Part model, mm, in its own coordinate system. Coordinates: 2 decimals unless noted, no trailing zeros. Write each loop counter-clockwise with the first axis right and the second up, starting at its lowest first coordinate (ties: lowest second). Pieces come first, ordered by that corner, then holes. Notation, with made-up numbers: (65, -23) -> (71, -23) arc R27 cw to (71, 0) -> close; hole circle Ø2 at (75.5, 1.25). An arc over 180 degrees is marked (long way). One line per question, with ' | ' between items. Start each with the question number.
Item 1: Two-plate mould, pull along X, no slides. Class faces 1 (the flat face through (-1, 6, 5)), 2 (the flat face through (-29.739, -1, 2)), 3 (the cylindrical face through (5.31, -0.76, 2.46)): pulls with the +X half, pulls with the -X half, needs draft (parallel to the pull), parting line crosses it, or undercut.
Item 2: Saw through at B-B (z = 1.4). Count the separate pieces of the cut face and the enclosed holes in it, and give its area (3 significant figures).
Item 3: Saw through at A-A (x = -7). List the corners of the cut face in (y, z).
Item 4: Saw through at C-C (x = 6.3). List the corners of the cut face in (y, z).
Item 5: Pin check, flat tips, straight feed: pin 1 (21 mm diameter, centred on x = -7, y = 0, fed in from -Z); pin 2 (2 mm diameter, centred on x = 18, y = 20.5, fed in from +Z). Stop position of each tip, or through.
Item 6: Probe probe 1 along Y at (x, z) = (-18, 3.45); probe 2 along Y at (x, z) = (-20.3, 1.6); probe 3 along X at (y, z) = (20, 4.2). List the from-to ranges inside material, lowest first. Write a range as [from, to].
from build123d import *

# Parameters (mm, degrees)
CROQUIS1_W              = 59
CROQUIS1_H              = 51
CROQUIS1_R              = 1.25
CROQUIS1_R_2            = 1.3
CROQUIS1_R_3            = 6.5
SALIENTE_EXTRUIR1_DEPTH = 5


with BuildPart() as part:
    # Croquis1 → Saliente-Extruir1 (new body)
    with BuildSketch(Plane.XY):
        with Locations((-0.238863052, -0.247607665)):
            Rectangle(CROQUIS1_W, CROQUIS1_H)
        with Locations((24.261136948, -17.747607665)):
            Circle(CROQUIS1_R, mode=Mode.SUBTRACT)
        with Locations((-18, 20.5)):
            Circle(CROQUIS1_R, mode=Mode.SUBTRACT)
        with Locations((18, 20.5)):
            Circle(CROQUIS1_R, mode=Mode.SUBTRACT)
        with Locations((-23, 20.5)):
            Circle(CROQUIS1_R_2, mode=Mode.SUBTRACT)
        with Locations((23, 20.5)):
            Circle(CROQUIS1_R_2, mode=Mode.SUBTRACT)
        with Locations((-7, 0)):
            Circle(CROQUIS1_R_3, mode=Mode.SUBTRACT)
        with Locations((-20.3, 0)):
            Circle(CROQUIS1_R, mode=Mode.SUBTRACT)
        with Locations((6.3, 0)):
            Circle(CROQUIS1_R, mode=Mode.SUBTRACT)
    extrude(amount=SALIENTE_EXTRUIR1_DEPTH)


solid = part.part
From the geometry:
1) face 1: needs draft | face 2: pulls with the -X half | face 3: undercut
2) separate pieces: 1 | enclosed holes: 8 | area: 2,840 mm2
3) outline: (-25.75, 0) -> (-6.5, 0) -> (-6.5, 5) -> (-25.75, 5) -> close; (6.5, 0) -> (25.25, 0) -> (25.25, 5) -> (6.5, 5) -> close
4) outline: (-25.75, 0) -> (-1.25, 0) -> (-1.25, 5) -> (-25.75, 5) -> close; (1.25, 0) -> (25.25, 0) -> (25.25, 5) -> (1.25, 5) -> close
5) pin 1: z = 0 | pin 2: through
6) probe 1: [-25.75, 19.25], [21.75, 25.25] | probe 2: [-25.75, -1.25], [1.25, 25.25] | probe 3: [-29.74, -24.2], [-21.8, -19.15], [-16.85, 16.85], [19.15, 21.8], [24.2, 29.26]
